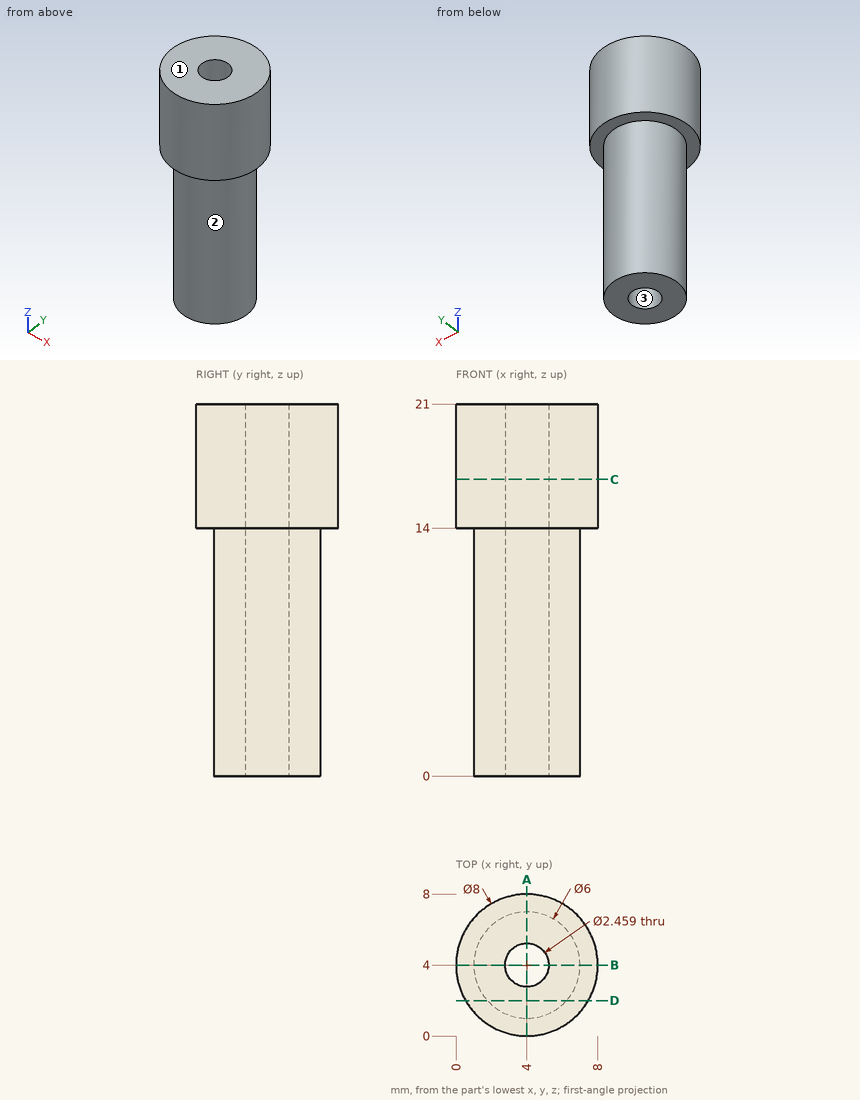
Here's the drawing with two shaded views (mm, measured from the low corner). I have some questions. Round coordinates to 2 decimals unless told otherwise and drop trailing zeros. Loops run counter-clockwise (first coordinate to the right, second up) from the corner with the lowest first, then second, coordinate; pieces in that order, holes last.
Item 1: Suppose I cut it at C-C, the plane z = 16.75. Write out the boundary of the cut face in (x, y).
Item 2: Suppose I cut it at A-A, the plane x = 4. Write out the boundary of the cut face in (y, z).
Item 3: Please list where these lines run through material, in increasing order: L1, parallel to Y at x = 4, z = 12.75; L2, parallel to Y at x = 4, z = 16; L3, parallel to Z at x = 1, y = 2.5.
Item 4: Suppose I cut it at D-D, the plane y = 2. Write out the boundary of the cut face in (x, z).
Item 5: If we mould it in two halves opening along Y, with no side actions, what happens to the marked faces 1, 2 and 3? For each: +Y half, -Y half, draft (parallel to the pull), parting line (faces both ways), or undercut.
Item 6: Will these pins go through, and if not, where does the flat tip stop? pin 1 Ø1.5 at (y, z) = (6.5, 7) entering from -X; pin 2 Ø1 at (x, z) = (3.5, 8.5) entering from +Y; pin 3 Ø3 at (x, z) = (5, 11) entering from -Y.
Reported:
1. outline: circle Ø8 at (4, 4); hole circle Ø2.46 at (4, 4)
2. outline: (0, 14) - (1, 14) - (1, 0) - (2.77, 0) - (2.77, 21) - (0, 21) - close; (5.23, 0) - (7, 0) - (7, 14) - (8, 14) - (8, 21) - (5.23, 21) - close
3. L1: y = 1 to 2.77, 5.23 to 7
3. L2: y = 0 to 2.77, 5.23 to 8
3. L3: z = 14 to 21
4. outline: (0.54, 14) - (1.76, 14) - (1.76, 0) - (6.24, 0) - (6.24, 14) - (7.46, 14) - (7.46, 21) - (0.54, 21) - close
5. face 1: draft
5. face 2: parting line
5. face 3: undercut
6. pin 1: stops at x = 1.56
6. pin 2: stops at y = 7
6. pin 3: stops at y = 1
